Source: CAD feature listing. Evaluate the final solid. Frame: model axes, mm. Coordinates: 2 decimals unless noted, no trailing zeros. Order: outer loops, then holes, each group sorted by start corner. A loop starts at its lowest first (then second) coordinate and runs counter-clockwise, first axis right, second up. Notation, with made-up numbers: (79.25, -0.75) - (89.25, -0.75) arc R31 cw to (89.25, 37.25) - close; hole circle Ø3 at (67, -4.5). An arc over 180 degrees is marked (long way). One line per question, with ' | ' between items. Start each with the question number.
(1) Draft query along Y for faces 1 (the flat face through (153, -25, 0)), 2 (the cylindrical face through (-852.14, -32.43, 9.39)), 3 (the flat face through (186.202, -411.559, 9.392)), 4 (the flat face through (188.604, 350.441, 9.392)). Return one class per face: +Y half, -Y half, draft (parallel to the pull), parting line (faces both ways), or undercut.
(2) Section B-B (y = 358.5). Return the cut outline in (x, z).
(3) Contact query for flat-ended pins moving along their axis: P1, Ø6, axis at x = -107.5, z = 14, coming from the -Y side; P2, Ø5.5, axis at x = -837.5, z = 12.5, coming from the +Y side; P3, Ø3, axis at y = -251.5, z = 8.5, coming from the -X side; P4, Ø3, axis at x = 395.5, y = -250.5, coming from the -Z side. Output: stop coordinate, or through.
(4) Section C-C (z = 5.5). Count the separate pieces of the cut face and the enclosed holes in it, then the cut area to 3 significant figures.
(5) Line query: line 1 along Y through (x, z) = (310, 14.75); line 2 along Y through (x, z) = (478, 15); line 3 along X through (y, z) = (82.5, 11.5) (3 decimals). Output: solid intervals per line, ascending.
(6) Section A-A (x = -164.5). Return the cut outline in (y, z).
from build123d import *

# Parameters (mm, degrees)
F0_W     = 38.1
F0_H     = 19.05
F0_W_2   = 152.4
F0_H_2   = 19.416131
F0_R     = 9.525
F0_W_3   = 50.8
F0_R_2   = 30.1244
F0_W_4   = 37.285626
F0_W_5   = 152.91512
F0_H_3   = 18.948435
F1_DEPTH = 19.05


with BuildPart() as f1:
    # F0 (on Top) → F1 (new body)
    with BuildSketch(Plane.XY):
        Polygon((273.206008, -643.359119), (578.006008, -643.359119), (578.006008, -186.159119), (578.006008, -167.109119), (578.006008, -160.759119), (476.885, -160.759119), (426.085, -160.759119), (101.6, -160.759119), (101.6, -186.159119), align=None)
        with Locations((304.956008, -608.434119)):
            Rectangle(F0_W, F0_H, mode=Mode.SUBTRACT)
        with Locations((304.956008, -544.934119)):
            Rectangle(F0_W, F0_H, mode=Mode.SUBTRACT)
        with Locations((419.256008, -608.251053)):
            Rectangle(F0_W_2, F0_H_2, mode=Mode.SUBTRACT)
        with Locations((533.556008, -608.434119)):
            Rectangle(F0_W, F0_H, mode=Mode.SUBTRACT)
        with Locations((419.256008, -544.567988)):
            Rectangle(F0_W_2, F0_H, mode=Mode.SUBTRACT)
        with Locations((533.556008, -544.934119)):
            Rectangle(F0_W, F0_H, mode=Mode.SUBTRACT)
        with Locations((451.006008, -382.642988)):
            Circle(F0_R, mode=Mode.SUBTRACT)
        Polygon((-914.4, -186.159119), (101.6, -186.159119), (101.6, -160.759119), (101.6, -43.478698), (92.075, -43.478698), (92.075, -24.428698), (101.6, -24.428698), (101.6, 93.240881), (50.8, 93.240881), (50.8, 74.190881), (0, 74.190881), (0, 93.240881), (-375.285, 93.240881), (-375.285, 74.190881), (-426.085, 74.190881), (-426.085, 93.240881), (-801.37, 93.240881), (-801.37, 74.190881), (-852.17, 74.190881), (-852.17, 93.240881), (-914.4, 93.240881), (-914.4, 74.190881), (-914.4, -167.109119), align=None)
        with Locations((-826.77, -151.234119)):
            Rectangle(F0_W_3, F0_H, mode=Mode.SUBTRACT)
        with Locations((-822.0456, -33.759119)):
            Circle(F0_R_2, mode=Mode.SUBTRACT)
        with Locations((-400.685, -151.234119)):
            Rectangle(F0_W_3, F0_H, mode=Mode.SUBTRACT)
        with Locations((-208.684325, -84.559119)):
            Circle(F0_R, mode=Mode.SUBTRACT)
        Polygon((-41.275, -24.428698), (-41.275, -33.953698), (-41.275, -43.478698), (-60.325, -43.478698), (-60.325, -33.953698), (-60.325, -24.428698), align=None, mode=Mode.SUBTRACT)
        with Locations((25.4, -151.234119)):
            Rectangle(F0_W_3, F0_H, mode=Mode.SUBTRACT)
        Polygon((-27.94, -78.209119), (24.7487, -78.209119), (73.66, -78.209119), (73.66, -116.309119), (-27.94, -116.309119), align=None, mode=Mode.SUBTRACT)
        Polygon((-25.4, -24.428698), (24.7487, -24.428698), (76.2, -24.428698), (76.2, -43.478698), (24.7487, -43.478698), (-25.4, -43.478698), (-25.4, -33.953698), align=None, mode=Mode.SUBTRACT)
        with Locations((-208.684325, 17.040881)):
            Circle(F0_R, mode=Mode.SUBTRACT)
        Polygon((-27.94, 10.690881), (-27.94, 48.790881), (73.66, 48.790881), (73.66, 10.690881), (24.7487, 10.690881), align=None, mode=Mode.SUBTRACT)
        Polygon((476.885, -160.759119), (578.006008, -160.759119), (578.006008, 74.190881), (578.006008, 93.240881), (476.885, 93.240881), (476.885, 74.190881), (426.085, 74.190881), (426.085, 93.240881), (101.6, 93.240881), (101.6, -24.428698), (111.125, -24.428698), (111.125, -43.478698), (101.6, -43.478698), (101.6, -160.759119), (426.085, -160.759119), (426.085, -141.709119), (476.885, -141.709119), align=None)
        Polygon((476.885, 93.240881), (578.006008, 93.240881), (578.006008, 575.840881), (273.206008, 575.840881), (101.6, 118.640881), (101.6, 93.240881), (426.085, 93.240881), align=None)
        with Locations((304.848075, 477.415881)):
            Rectangle(F0_W_4, F0_H, mode=Mode.SUBTRACT)
        with Locations((304.956008, 540.915881)):
            Rectangle(F0_W, F0_H, mode=Mode.SUBTRACT)
        with Locations((418.998448, 477.466663)):
            Rectangle(F0_W_5, F0_H_3, mode=Mode.SUBTRACT)
        with Locations((533.556008, 477.415881)):
            Rectangle(F0_W, F0_H, mode=Mode.SUBTRACT)
        with Locations((419.256008, 540.915881)):
            Rectangle(F0_W_2, F0_H, mode=Mode.SUBTRACT)
        with Locations((533.556008, 540.915881)):
            Rectangle(F0_W, F0_H, mode=Mode.SUBTRACT)
        Polygon((-914.4, 118.640881), (-914.4, 93.240881), (-852.17, 93.240881), (-801.37, 93.240881), (-426.085, 93.240881), (-375.285, 93.240881), (0, 93.240881), (50.8, 93.240881), (101.6, 93.240881), (101.6, 118.640881), align=None)
    extrude(amount=F1_DEPTH)


solid = f1.part
Response values:
1) face 1: draft | face 2: undercut | face 3: -Y half | face 4: +Y half
2) outline: (191.63, 0) - (578.01, 0) - (578.01, 19.05) - (191.63, 19.05) - close
3) P1: stops at y = -186.16 | P2: stops at y = 118.64 | P3: stops at x = 125.56 | P4: stops at z = 0
4) separate pieces: 1 | enclosed holes: 29 | area: 773,000 mm²
5) line 1: y = -643.36 to -617.96, -598.91 to -554.46, -535.41 to 467.89, 486.94 to 531.39, 550.44 to 575.84 | line 2: y = -643.36 to -617.96, -598.54 to -554.09, -535.04 to 467.99, 486.94 to 531.39, 550.44 to 575.84 | line 3: x = -914.4 to -852.17, -801.37 to -426.085, -375.285 to 0, 50.8 to 426.085, 476.885 to 578.006
6) outline: (-186.16, 0) - (118.64, 0) - (118.64, 19.05) - (-186.16, 19.05) - close
